CAD build for the part. Positions are in the model's coordinates, mm. Face numbers are marked on the shaded views. A direction names the side the tool comes from. Round coordinates to 2 decimals unless told otherwise and drop trailing zeros. Loops run counter-clockwise (first coordinate to the right, second up) from the corner with the lowest first, then second, coordinate; pieces in that order, holes last. Notation, with made-up numbers: M 14,71 L 58,71 A19 ccw 58,105 Z; hole C -15.75,88 d6. An arc over 180 degrees is marked long. Use a Markdown table: item, result. Add a question column.
(1) Band-saw the part on A-A, the plane z = 3. Write the cut outline in (x, y), and give its area (3 significant figures).
(2) Band-saw the part on B-B, the plane x = 0. Write the cut outline in (y, z), and give its area (3 significant figures).
(3) Band-saw the part on D-D, the plane y = 3. Write the cut outline in (x, z).
(4) Which spindle directions (+Z, -Z, +X, -X, +Y, -Y) get a long thin tool onto all of the face, cutting with end or side? Do the marked faces 1 and 2. Say none if no direction does.
(5) Flat gauge pin, fed straight in: P1, Ø6, axis at x = 5.5, y = -5, coming from the -Z side. Where does the tip first touch, or does it go through?
(6) Wall check: L1, parallel to Y at x = 7.25, z = 14.75; L2, parallel to Z at x = 0.25, y = 1.75; L3, parallel to Z at x = 9, y = 1.5. Give the ranges that are in metal, low to high.
(7) Two-plate mould, pull along X, no slides. Class the marked faces 3, 4 and 5: released by +X, released by -X, zero draft, split by the parting line, or undercut.
(8) Band-saw the part on C-C, the plane y = -10.5. Write the cut outline in (x, z), and give its area (3 significant figures).
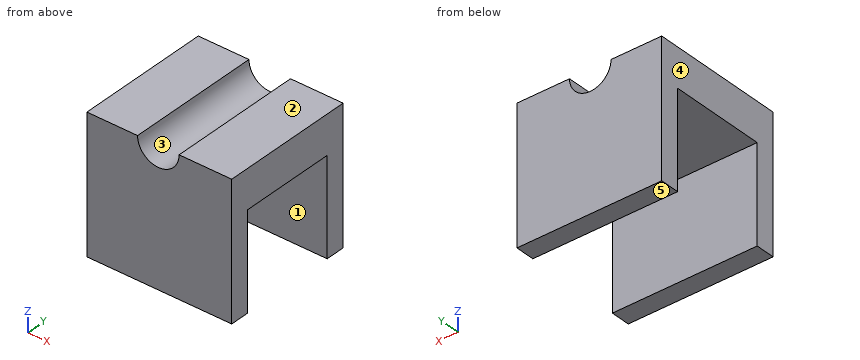
from build123d import *

# Parameters (mm, degrees)
F0_W     = 30
F0_H     = 28
F1_DEPTH = 28
F3_DEPTH = 28.001
F4_W     = 30
F4_H     = 20
F5_DEPTH = 20


with BuildPart() as f1:
    # F0 (on Top) → F1 (new body)
    with BuildSketch(Plane.XY):
        with Locations((0.2024, 0.448397)):
            Rectangle(F0_W, F0_H)
    extrude(amount=F1_DEPTH)

    # F2 (on face) → F3 (cut, through all)
    with BuildSketch(Plane.XZ.offset(13.551603)):
        with BuildLine():
            ThreePointArc((-4.3, 28), (0, 23.7), (4.3, 28))
            Line((4.3, 28), (-4.3, 28))
        make_face()
    extrude(amount=-F3_DEPTH, mode=Mode.SUBTRACT)

    # F4 (on face) → F5 (cut)
    with BuildSketch(Plane(origin=(0, 0, 0), x_dir=(1, 0, 0), z_dir=(0, 0, -1))):
        with Locations((0.2024, -0.448397)):
            Rectangle(F4_W, F4_H)
    extrude(amount=-F5_DEPTH, mode=Mode.SUBTRACT)


solid = f1.part
Return value:
| question | item | result |
|---|---|---|
| 1 | outline | M -14.8,-13.55 L 15.2,-13.55 L 15.2,-9.55 L -14.8,-9.55 Z; M -14.8,10.45 L 15.2,10.45 L 15.2,14.45 L -14.8,14.45 Z |
| 1 | area | 240 mm^2 |
| 2 | outline | M -13.55,0 L -9.55,0 L -9.55,20 L 10.45,20 L 10.45,0 L 14.45,0 L 14.45,23.7 L -13.55,23.7 Z |
| 2 | area | 264 mm^2 |
| 3 | outline | M -14.8,20 L 15.2,20 L 15.2,28 L 4.3,28 A4.3 cw -4.3,28 L -14.8,28 Z |
| 4 | face 1 | -Z, +X, -X |
| 4 | face 2 | +Z, +X, -X, +Y, -Y |
| 5 | P1 | z = 20 |
| 6 | L1 | -13.55 to -9.55, 10.45 to 14.45 |
| 6 | L2 | 20 to 23.71 |
| 6 | L3 | 20 to 28 |
| 7 | face 3 | undercut |
| 7 | face 4 | released by -X |
| 7 | face 5 | zero draft |
| 8 | outline | M -14.8,0 L 15.2,0 L 15.2,28 L 4.3,28 A4.3 cw -4.3,28 L -14.8,28 Z |
| 8 | area | 811 mm^2 |
